Geometry: final body of the model. Coordinates: model frame, mm. A direction names the side the tool comes from. Give positions to 0.01 mm unless a question says otherwise; leave off trailing zeros. Loops run counter-clockwise (first coordinate to the right, second up) from the corner with the lowest first, then second, coordinate; pieces in that order, holes last.
1. Draft query along Y for faces 1 (the face through (36.7, -72.2, 19.1)), 2 (the face through (23, -39, 1)), 3 (the face through (37, -52, 18.4)). Return one class per face: +Y half, -Y half, draft (parallel to the pull), parting line (faces both ways), or undercut.
2. Section C-C, the plane z = 12. Output: boundary loops of the cut face in (x, y).
3. Section A-A, the plane y = -63. State how many separate pieces and enclosed holes the cut face has, then the cut area to 3 significant figures.
4. Section D-D, the plane y = -76. Output: boundary loops of the cut face in (x, z).
5. Material intervals for line 1 along X through (y, z) = (-34, 3.75); line 2 along Z through (x, y) = (9.5, -73); line 3 along X through (y, z) = (-18.5, 12.5), sorted ascending.
6. First-contact query: P1, Ø18.5, axis at x = 26.5, y = -45, coming from the +Z side; P2, Ø9, axis at y = -63, z = 9.8, coming from the +X side; P3, Ø1.3, axis at y = -55, z = 0.5, coming from the +X side; P4, Ø12, axis at x = 20, z = 13.5, coming from the -Y side. Flat tips, straight axial feed; report the tip coordinate or a pass-through.
7. Section B-B, the plane x = 23. Output: boundary loops of the cut face in (y, z), then the cut area to 3 significant figures.
8. Access query for faces 4 (the face through (9, -70, 18.4)), 5 (the face through (22, -114, 1)), 6 (the face through (13.1, -71, 10)), 7 (the face through (12.367, -8.396, 4.136)), 8 (the face through (23, -87, 1)). Directions: +Z, -Z, +X, -X, +Y, -Y. A direction counts if a zero-diameter tool reaches every point of the face in a straight line with its end or side. Return the directions, or none.
from build123d import *

# Parameters (mm, degrees)
F1_DEPTH = 114
F3_DEPTH = 25
F5_DEPTH = 5
F6_R     = 4
F7_DEPTH = 30
F9_DEPTH = 5


with BuildPart() as f1:
    # F0 (on Front) → F1 (new body)
    with BuildSketch(Plane.XZ):
        with BuildLine():
            ThreePointArc((-11.5, 3.2), (-10.5627416998, 0.9372583002), (-8.3, 0))
            Line((-8.3, 0), (0, 0))
            Line((0, 0), (8.3, 0))
            ThreePointArc((8.3, 0), (10.5627416998, 0.9372583002), (11.5, 3.2))
            Line((11.5, 3.2), (11.5, 16.8))
            ThreePointArc((11.5, 16.8), (11.9686291501, 17.9313708499), (13.1, 18.4))
            Line((13.1, 18.4), (15.9, 18.4))
            Line((15.9, 18.4), (15.9, 20))
            Line((15.9, 20), (13.1, 20))
            ThreePointArc((13.1, 20), (10.8372583002, 19.0627416998), (9.9, 16.8))
            Line((9.9, 16.8), (9.9, 3.2))
            ThreePointArc((9.9, 3.2), (9.4313708499, 2.0686291501), (8.3, 1.6))
            Line((8.3, 1.6), (0, 1.6))
            Line((0, 1.6), (-8.3, 1.6))
            ThreePointArc((-8.3, 1.6), (-9.4313708499, 2.0686291501), (-9.9, 3.2))
            Line((-9.9, 3.2), (-9.9, 16.8))
            ThreePointArc((-9.9, 16.8), (-10.8372583002, 19.0627416998), (-13.1, 20))
            Line((-13.1, 20), (-15.9, 20))
            Line((-15.9, 20), (-15.9, 18.4))
            Line((-15.9, 18.4), (-13.1, 18.4))
            ThreePointArc((-13.1, 18.4), (-11.9686291501, 17.9313708499), (-11.5, 16.8))
            Line((-11.5, 16.8), (-11.5, 3.2))
        make_face()
    extrude(amount=F1_DEPTH)

    # F2 (on face) → F3 (cut)
    with BuildSketch(Plane.XY.offset(1.6)):
        with BuildLine():
            ThreePointArc((-7, -46), (0, -53), (7, -46))
            Line((7, -46), (-7, -46))
        make_face()
        with BuildLine():
            Line((-7, -46), (7, -46))
            ThreePointArc((7, -46), (0, -39), (-7, -46))
        make_face()
        with BuildLine():
            Line((7, -80), (7, -46))
            ThreePointArc((7, -46), (0, -53), (-7, -46))
            Line((-7, -46), (-7, -80))
            ThreePointArc((-7, -80), (0, -73), (7, -80))
        make_face()
        with BuildLine():
            ThreePointArc((-7, -80), (0, -87), (7, -80))
            Line((7, -80), (-7, -80))
        make_face()
        with BuildLine():
            Line((-7, -80), (7, -80))
            ThreePointArc((7, -80), (0, -73), (-7, -80))
        make_face()
    extrude(amount=-F3_DEPTH, mode=Mode.SUBTRACT)

    # F4 (on face) → F5 (cut)
    with BuildSketch(Plane.XY.offset(20)):
        Polygon((-11.5, 0), (-15.9, 0), (-15.9, -55), align=None)
        Polygon((-11.5, -74.4), (-15.9, -70), (-15.9, -114), (-11.5, -114), align=None)
    extrude(amount=-F5_DEPTH, mode=Mode.SUBTRACT)

    # F6 (on face) → F7 (cut)
    with BuildSketch(Plane.YZ.offset(11.5)):
        with Locations((-63, 9.8)):
            Circle(F6_R)
    extrude(amount=-F7_DEPTH, mode=Mode.SUBTRACT)

    # F8 (on face) → F9 (cut, symmetric)
    with BuildSketch(Plane.YZ.offset(11.5)):
        with BuildLine():
            Line((-38.3930956715, 27.5), (-15.5696902422, 8.348888922))
            ThreePointArc((-15.5696902422, 8.348888922), (-8.0505035831, 4.0076844804), (0.5, 2.5))
            Line((0.5, 2.5), (5, 2.5))
            Line((5, 2.5), (5, 27.5))
            Line((5, 27.5), (-38.3930956715, 27.5))
        make_face()
    extrude(amount=F9_DEPTH, both=True, mode=Mode.SUBTRACT)


with BuildPart() as f10_1:
    # F10: instance of F1
    add(f1.part.mirror(Plane.YZ.offset(11.5)))


solid = f10_1.part
Answers below:
1. face 1: -Y half
1. face 2: undercut
1. face 3: draft
2. outline: (11.5, -114) - (13.1, -114) - (13.1, -66.34) - (11.5, -66.34) - close; (11.5, -59.66) - (13.1, -59.66) - (13.1, -19.92) - (11.5, -19.92) - close; (32.9, -114) - (34.5, -114) - (34.5, -66.34) - (32.9, -66.34) - close; (32.9, -59.66) - (34.5, -59.66) - (34.5, 0) - (32.9, 0) - close
3. separate pieces: 4
3. enclosed holes: 0
3. area: 55.2 mm2
4. outline: (7.1, 18.4) - (9.9, 18.4) arc R1.6 cw to (11.5, 16.8) - (11.5, 3.2) arc R3.2 ccw to (14.7, 0) - (16, 0) - (16, 1.6) - (14.7, 1.6) arc R1.6 cw to (13.1, 3.2) - (13.1, 16.8) arc R3.2 ccw to (9.9, 20) - (7.1, 20) - close; (30, 0) - (31.3, 0) arc R3.2 ccw to (34.5, 3.2) - (34.5, 19.57) arc R3.2 ccw to (32.9, 16.8) - (32.9, 3.2) arc R1.6 cw to (31.3, 1.6) - (30, 1.6) - close
5. line 1: x = 11.5 to 13.1, 32.9 to 34.5
5. line 2: z = 18.4 to 20
5. line 3: x = 32.9 to 34.5
6. P1: stops at z = 19.98
6. P2: stops at x = 34.5
6. P3: stops at x = 33.76
6. P4: passes through
7. outline: (-114, 0) - (-87, 0) - (-87, 1.6) - (-114, 1.6) - close; (-39, 0) - (0, 0) - (0, 1.6) - (-39, 1.6) - close
7. area: 106 mm2
8. face 4: -Z, -X, +Y, -Y
8. face 5: +Z, -Z, +X, -X, -Y
8. face 6: +Z, +Y, -Y
8. face 7: +Z, -X, +Y
8. face 8: +Z, -Z
